Build history of the part. All positions in model axes, mm. Face numbers are marked on the shaded views. A direction names the side the tool comes from. Give positions to 0.01 mm unless a question says otherwise; leave off trailing zeros. Write each loop counter-clockwise with the first axis right and the second up, starting at its lowest first coordinate (ties: lowest second). Pieces come first, ordered by that corner, then holes.
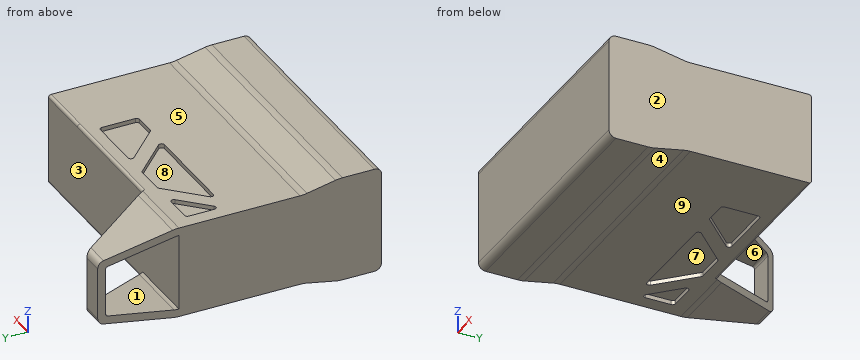
from build123d import *

# Parameters (mm, degrees)
EXTRUDE_2_DEPTH        = 140
SKETCH_7_W             = 65
SKETCH_7_H             = 74.928349175
CUT_EXTRUDE_2_DEPTH    = 150
CUT_EXTRUDE_3_DEPTH    = 150
FILLET_1_R             = 2
FILLET_2_R             = 2
CUT_EXTRUDE_4_DEPTH    = 3
FILLET_3_R             = 2
FILLET_3_OF_MIRROR_1_R = 2
EXTRUDE_3_DEPTH        = 40


with BuildPart() as part:
    # 草图2 → 凸台-拉伸2 (new body)
    with BuildSketch(Plane(origin=(0, 0, 0), x_dir=(0, 0, -1), z_dir=(1, 0, 0))):
        with BuildLine():
            Line((37.5, -95.110619623), (37.5, -72.586107463))
            ThreePointArc((37.5, -72.586107463), (37.378333167, -70.122667014), (37.014516892, -67.683204084))
            Line((37.014516892, -67.683204084), (32.985483108, -47.538035162))
            ThreePointArc((32.985483108, -47.538035162), (32.621666833, -45.098572232), (32.5, -42.635131783))
            Line((32.5, -42.635131783), (32.5, 42.635131783))
            ThreePointArc((32.5, 42.635131783), (32.398982849, 44.880271666), (32.096747752, 47.107267738))
            Line((32.096747752, 47.107267738), (23.246467783, 95.783807568))
            ThreePointArc((23.246467783, 95.783807568), (21.530855429, 98.728139028), (18.327118233, 99.889380377))
            Line((18.327118233, 99.889380377), (-18.327118233, 99.889380377))
            ThreePointArc((-18.327118233, 99.889380377), (-21.530855429, 98.728139028), (-23.246467783, 95.783807568))
            Line((-23.246467783, 95.783807568), (-32.096747752, 47.107267738))
            ThreePointArc((-32.096747752, 47.107267738), (-32.398982849, 44.880271666), (-32.5, 42.635131783))
            Line((-32.5, 42.635131783), (-32.5, -42.635131783))
            ThreePointArc((-32.5, -42.635131783), (-32.621666833, -45.098572232), (-32.985483108, -47.538035162))
            Line((-32.985483108, -47.538035162), (-37.014516892, -67.683204084))
            ThreePointArc((-37.014516892, -67.683204084), (-37.378333167, -70.122667014), (-37.5, -72.586107463))
            Line((-37.5, -72.586107463), (-37.5, -95.110619623))
            ThreePointArc((-37.5, -95.110619623), (-36.035533906, -98.646153529), (-32.5, -100.110619623))
            Line((-32.5, -100.110619623), (32.5, -100.110619623))
            ThreePointArc((32.5, -100.110619623), (36.035533906, -98.646153529), (37.5, -95.110619623))
        make_face()
    extrude(amount=EXTRUDE_2_DEPTH)

    # 草图7 → 切除-拉伸2 (cut, along a direction that is not the sketch's normal)
    with BuildSketch(Plane(origin=(55.371135265, 33.848837106, 0), x_dir=(0, 0, -1), z_dir=(0.853206949, 0.521572529, 0))):
        with Locations((0, 47.762138861)):
            Rectangle(SKETCH_7_W, SKETCH_7_H)
    extrude(amount=CUT_EXTRUDE_2_DEPTH, dir=(1, 0, 0), mode=Mode.SUBTRACT)

    # 草图8 → 切除-拉伸3 (cut)
    with BuildSketch(Plane.ZY):
        with BuildLine():
            Line((17.909830056, 94.389380377), (-17.909830056, 94.389380377))
            Line((-17.909830056, 94.389380377), (-26.685463247, 46.123397828))
            ThreePointArc((-26.685463247, 46.123397828), (-26.921206622, 44.386340892), (-27, 42.635131783))
            Line((-27, 42.635131783), (27, 42.635131783))
            ThreePointArc((27, 42.635131783), (26.921206622, 44.386340892), (26.685463247, 46.123397828))
            Line((26.685463247, 46.123397828), (17.909830056, 94.389380377))
        make_face()
    extrude(amount=-CUT_EXTRUDE_3_DEPTH, mode=Mode.SUBTRACT)

    # 圆角1
    fillet_1_edges = [part.edges().sort_by_distance(p)[0] for p in [
        (9.181097951, 94.389380377, 17.909830056),
        (9.181097951, 94.389380377, -17.909830056),
    ]]
    fillet(fillet_1_edges, radius=FILLET_1_R)

    # 圆角2
    fillet_2_edges = [part.edges().sort_by_distance(p)[0] for p in [
        (95, 42.635131783, 32.5),
        (95, 42.635131783, -32.5),
    ]]
    fillet(fillet_2_edges, radius=FILLET_2_R)

    # 草图9 → 切除-拉伸4 (cut)
    with BuildSketch(Plane(origin=(0, 0, -32.5), x_dir=(-1, 0, 0), z_dir=(0, 0, -1))):
        Polygon((-85, 32.635131783), (-130, 32.635131783), (-130, 5), (-112.635131783, 5), align=None)
        Polygon((-49.142135624, 32.635131783), (-70.857864376, 32.635131783), (-98.492996159, 5), (-21.507003841, 5), align=None)
        Polygon((-10, 32.635131783), (-35, 32.635131783), (-10, 7.635131783), align=None)
    cut_extrude_4 = extrude(amount=-CUT_EXTRUDE_4_DEPTH, mode=Mode.SUBTRACT)

    # 圆角3
    fillet_3_edges = [part.edges().sort_by_distance(p)[0] for p in [
        (21.507003841, 5, -31),
        (98.492996159, 5, -31),
        (70.857864376, 32.635131783, -31),
        (49.142135624, 32.635131783, -31),
        (35, 32.635131783, -31),
        (10, 32.635131783, -31),
        (10, 7.635131783, -31),
        (85, 32.635131783, -31),
        (112.635131783, 5, -31),
        (130, 5, -31),
        (130, 32.635131783, -31),
    ]]
    fillet(fillet_3_edges, radius=FILLET_3_R)

    # 镜向1: 切除-拉伸4 across plane
    add(cut_extrude_4.mirror(Plane.XY), mode=Mode.SUBTRACT)

    # 圆角3 of 镜向1
    fillet_3_of_mirror_1_edges = [part.edges().sort_by_distance(p)[0] for p in [
        (21.507003841, 5, 31),
        (98.492996159, 5, 31),
        (70.857864376, 32.635131783, 31),
        (49.142135624, 32.635131783, 31),
        (35, 32.635131783, 31),
        (10, 32.635131783, 31),
        (10, 7.635131783, 31),
        (85, 32.635131783, 31),
        (112.635131783, 5, 31),
        (130, 5, 31),
        (130, 32.635131783, 31),
    ]]
    fillet(fillet_3_of_mirror_1_edges, radius=FILLET_3_OF_MIRROR_1_R)

    # 草图10 → 凸台-拉伸3 (add)
    with BuildSketch(Plane(origin=(140, 0, 0), x_dir=(0, 0, -1), z_dir=(1, 0, 0))):
        with BuildLine():
            Line((32.5, -42.635131783), (32.5, 40.635131783))
            ThreePointArc((32.5, 40.635131783), (31.914213562, 42.049345346), (30.5, 42.635131783))
            Line((30.5, 42.635131783), (-30.5, 42.635131783))
            ThreePointArc((-30.5, 42.635131783), (-31.914213562, 42.049345346), (-32.5, 40.635131783))
            Line((-32.5, 40.635131783), (-32.5, -42.635131783))
            ThreePointArc((-32.5, -42.635131783), (-32.621666833, -45.098572232), (-32.985483108, -47.538035162))
            Line((-32.985483108, -47.538035162), (-37.014516892, -67.683204084))
            ThreePointArc((-37.014516892, -67.683204084), (-37.378333167, -70.122667014), (-37.5, -72.586107463))
            Line((-37.5, -72.586107463), (-37.5, -95.110619623))
            ThreePointArc((-37.5, -95.110619623), (-36.035533906, -98.646153529), (-32.5, -100.110619623))
            Line((-32.5, -100.110619623), (32.5, -100.110619623))
            ThreePointArc((32.5, -100.110619623), (36.035533906, -98.646153529), (37.5, -95.110619623))
            Line((37.5, -95.110619623), (37.5, -72.586107463))
            ThreePointArc((37.5, -72.586107463), (37.378333167, -70.122667014), (37.014516892, -67.683204084))
            Line((37.014516892, -67.683204084), (32.985483108, -47.538035162))
            ThreePointArc((32.985483108, -47.538035162), (32.621666833, -45.098572232), (32.5, -42.635131783))
        make_face()
    extrude(amount=EXTRUDE_3_DEPTH)


solid = part.part
(1) 3-axis set-ups, long thin cutter, end or side, ignore diameter. For the marked faces 5, 6, 7, 8 and 9: which of +Z, -Z, +X, -X, +Y, -Y reach the whole face in a straight line?
(2) Saw through at C-C, the plane x = 163. List the corners of the cut face in (y, z).
(3) Saw through at A-A, the plane z = 3.5. List the corners of the cut face in (x, y).
(4) Saw through at D-D, the plane y = -54. List the corners of the cut face in (x, z).
(5) Saw through at B-B, the plane y = 87. List the corners of the cut face in (x, z).
(6) Probe line 1 (Y direction, x = 150.5, z = 0); line 2 (Z direction, x = 41, y = 46.5); line 3 (Z direction, x = 117, y = 16). List the from-to ranges inside material, lowest first.
(7) Drop flat-ended pins along their axis: pin 1 (5 mm diameter, centred on x = 89, z = -20, fed in from +Y); pin 2 (22 mm diameter, centred on x = 115.5, y = 25.5, fed in from -Z); pin 3 (22 mm diameter, centred on x = 76.5, y = 25.5, fed in from +Z). Give the stop position or say it passes through.
(8) Mould opens along Z. For the marked faces 1, 2, 3 and 4 say: +Z half, -Z half, draft (parallel to the pull), parting line (faces both ways), or undercut.
Computed values:
1. face 5: +Z, +X, -X, +Y
1. face 6: +X, -X
1. face 7: -Z
1. face 8: +Z
1. face 9: -Z, +X, -X, +Y
2. outline: (-100.11, -32.5) arc R5 ccw to (-95.11, -37.5) - (-72.59, -37.5) arc R25 ccw to (-67.68, -37.01) - (-47.54, -32.99) arc R25 cw to (-42.64, -32.5) - (40.64, -32.5) arc R2 ccw to (42.64, -30.5) - (42.64, 30.5) arc R2 ccw to (40.64, 32.5) - (-42.64, 32.5) arc R25 cw to (-47.54, 32.99) - (-67.68, 37.01) arc R25 ccw to (-72.59, 37.5) - (-95.11, 37.5) arc R5 ccw to (-100.11, 32.5) - close
3. outline: (0, -100.11) - (180, -100.11) - (180, 42.64) - (0, 42.64) - close; (0, 94.39) - (18.36, 94.39) - (15, 99.89) - (0, 99.89) - close
4. outline: (0, -34.28) - (180, -34.28) - (180, 34.28) - (0, 34.28) - close
5. outline: (0, -24.84) - (22.88, -24.84) - (22.88, -19.25) - (0, -19.25) - close; (0, 19.25) - (22.88, 19.25) - (22.88, 24.84) - (0, 24.84) - close
6. line 1: y = -100.11 to 42.64
6. line 2: z = -32.2 to -26.62, 26.62 to 32.2
6. line 3: z = -29.5 to 29.5
7. pin 1: stops at y = 42.64
7. pin 2: stops at z = -32.5
7. pin 3: stops at z = 32.5
8. face 1: undercut
8. face 2: draft
8. face 3: undercut
8. face 4: -Z half
